Can you work these out from the model? Positions are in its coordinate system, mm. A direction names the side the tool comes from. Coordinates: 2 decimals unless noted, no trailing zeros. Loops run counter-clockwise (first coordinate to the right, second up) from the corner with the lowest first, then second, coordinate; pieces in that order, holes last. Notation, with made-up numbers: (-1.5, 40.5) -> (50.5, 40.5) arc R31 cw to (50.5, 70.5) -> close; hole circle Ø2 at (76, 73). An arc over 180 degrees is marked (long way). Put each result on its own line as item: value. Start each with the question number.
Item 1: For faces 5 (the flat face through (-0.167, 28.563, 2.995)), 6 (the flat face through (0.167, 28.563, -2.995)), 7 (the conical face through (-0.98, 4.273, 7.465)), 8 (the cylindrical face through (7.154, 19.806, 2.253)), 9 (the cylindrical face through (-4.864, 18.888, 4.461)), which set-ups out of +Z, -Z, +X, -X, +Y, -Y let a thin tool reach every point of the face, with its end or its side?
Item 2: If we section it at A-A on y = 25.5: Please give me the cut outline in (x, z).
Item 3: Will these pins go through, and if not, where does the flat tip stop? P1, Ø3, axis at x = 3, y = 19, coming from the -Z side; P2, Ø6, axis at x = 2, y = 24.5, coming from the -Z side; P3, Ø10.5, axis at x = -0.5, z = 1, coming from the -Y side.
Item 4: Please list where these lines run through material, in increasing order: L1, parallel to X at y = 17.75, z = 0; L2, parallel to Y at x = -9, z = -6.75. Write a range as from..to.
Item 5: We'd pull the mould along Y, two halves only. Please class faces 1 (the conical face through (9.038, 5.064, 2.846)), 2 (the conical face through (-7.57, 3.17, -5.8)), 3 (the flat face through (3, 23.1, 0)), 4 (the flat face through (-2.68, 28.56, 1.35)): pulls with the +Y half, pulls with the -Y half, needs draft (parallel to the pull), parting line crosses it, or undercut.
```python
from build123d import *

# Parameters (mm, degrees)
CASCA1_T                 = -0.9
RESSALTO_EXTRUS_O1_DEPTH = 9
FILETE1_R                = 1
ESBO_O3_R                = 2.38125
CORTE_EXTRUS_O1_DEPTH    = 34.0000001
ESQUISSE1_R              = 6.732461852
ENL_V_MAT_EXTRU_1_DEPTH  = 9


with BuildPart() as part:
    # Esboço1 → Revolução1 (revolve)
    with BuildSketch(Plane.XY):
        Polygon((0, 0), (13.5, 0), (8.5, 4), (14, 10), (7.5, 15), (7.5, 24), (0, 24), align=None)
    revolve(axis=Axis((0, 24, 0), (0, -1, 0)))

    # Casca1
    casca1_openings = [part.faces().sort_by_distance(p)[0] for p in [
        (-13.5, 0, 0),
    ]]
    offset(amount=CASCA1_T, openings=casca1_openings, kind=Kind.INTERSECTION)

    # Esboço2 → Ressalto-extrusão1 (add)
    with BuildSketch(Plane(origin=(0, 24, 0), x_dir=(1, 0, 0), z_dir=(0, 1, 0))):
        Polygon((2.496763598, 3.885808136), (-2.11682676, 4.105164771), (-4.613590359, 0.219356636), (-2.496763598, -3.885808136), (2.11682676, -4.105164771), (4.613590359, -0.219356636), align=None)
    extrude(amount=RESSALTO_EXTRUS_O1_DEPTH)

    # Filete1
    filete1_edges = [part.edges().sort_by_distance(p)[0] for p in [
        (-7.5, 15, 0),
        (-14, 10, 0),
        (-8.5, 4, 0),
    ]]
    fillet(filete1_edges, radius=FILETE1_R)

    # Esboço3 → Corte-extrusão1 (cut, through all)
    with BuildSketch(Plane(origin=(0, 33, 0), x_dir=(1, 0, 0), z_dir=(0, 1, 0))):
        Circle(ESBO_O3_R)
    extrude(amount=-CORTE_EXTRUS_O1_DEPTH, mode=Mode.SUBTRACT)

    # Esquisse1 → Enlèv. mat.-Extru.1 (cut)
    with BuildSketch(Plane(origin=(0, 33, 0), x_dir=(1, 0, 0), z_dir=(0, 1, 0))):
        Circle(ESQUISSE1_R)
        Polygon((1.58762007, -3.078873578), (3.460192769, -0.164517477), (1.872572699, 2.914356102), (-1.58762007, 3.078873578), (-3.460192769, 0.164517477), (-1.872572699, -2.914356102), align=None, mode=Mode.SUBTRACT)
    extrude(amount=-ENL_V_MAT_EXTRU_1_DEPTH, mode=Mode.SUBTRACT)


solid = part.part
```
Solutions:
1. face 5: +Z, -X, +Y
1. face 6: -Z, +X, +Y
1. face 7: none
1. face 8: +Y
1. face 9: -Y
2. outline: (-3.46, -0.16) -> (-1.59, -3.08) -> (1.87, -2.91) -> (3.46, 0.16) -> (1.59, 3.08) -> (-1.87, 2.91) -> close; hole circle Ø4.76 at (0, 0)
3. P1: z = -7.35
3. P2: z = -7.5
3. P3: y = 23.1
4. L1: -7.5..-6.6, 6.6..7.5
4. L2: 0.65..1.8, 7..8.33, 10.98..12.12
5. face 1: undercut
5. face 2: undercut
5. face 3: pulls with the -Y half
5. face 4: needs draft
